Study the drawing (mm; zero at the part's minimum x, y, z) and answer. A direction names the side the tool comes from. Coordinates: 2 decimals unless noted, no trailing zeros. Order: outer loops, then holes, each group sorted by start corner. A loop starts at its lowest first (then second) coordinate and runs counter-clockwise, first axis right, second up. Notation, with made-up numbers: (-0.75, 68) -> (17.25, 68) arc R13 cw to (17.25, 90) -> close; hole circle Ø9 at (30, 30). An arc over 180 degrees is marked (long way). Answer in a Markdown table with one row per item. Add a question column.
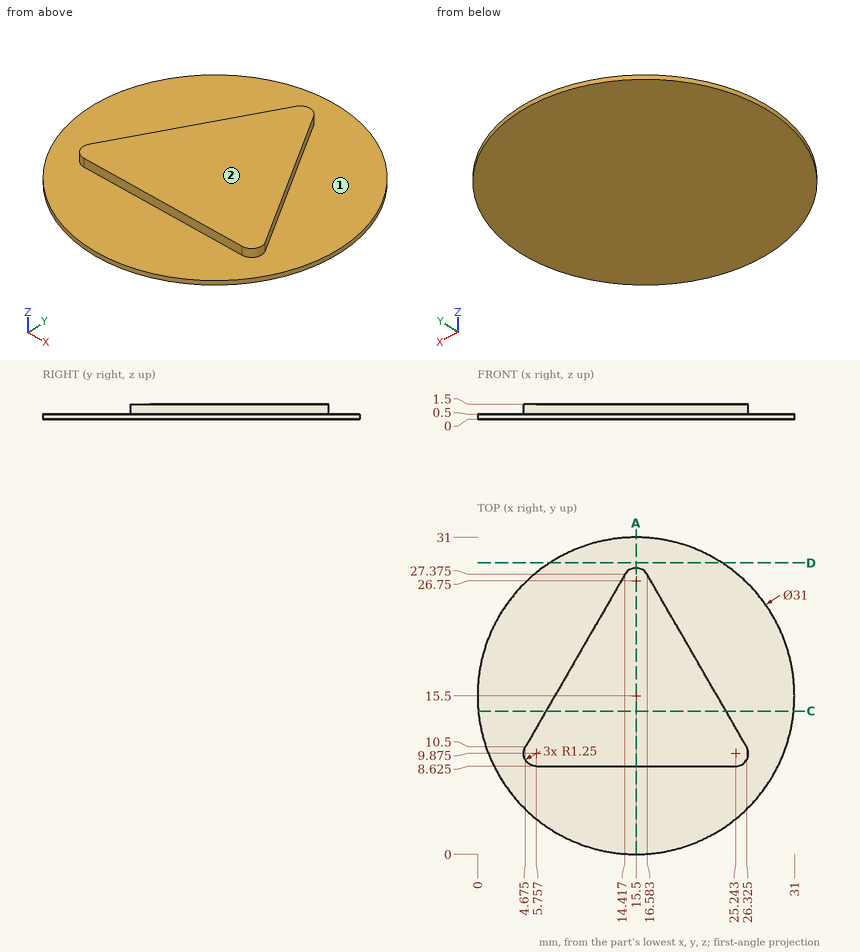
Q1. Straight lines are drawn through the part: line 1 (Z direction, x = 12.5, y = 4.5); line 2 (X direction, y = 10, z = 1); line 3 (Y direction, x = 11, z = 0.6) (1 decimal). For each, find the intervals that lie inside material, in ascending order.
Q2. A cutting plane is placed at A-A (x = 15.5). Determine the outline of the cut face in (y, z) (1 decimal).
Q3. Given pin 1 (0.8 mm diameter, centred on x = 12.5, z = 1, fed in from -Y) (3 decimals); pin 2 (4 mm diameter, centred on x = 25.5, y = 4.5, fed in from +Z), each flat-ended and moving along its own axis, determine where each tip first touches the part or whether it passes through.
Q4. A cutting plane is placed at D-D (y = 28.5). Determine the outline of the cut face in (x, z).
Q5. A cutting plane is placed at C-C (y = 14). Determine the outline of the cut face in (x, z) (1 decimal).
Q6. For the marked faces 1 and 2, determine the directions among +Z, -Z, +X, -X, +Y, -Y from which every point of the face is accessible in a straight line to the end or side of a thin tool.
Returned:
| question | item | result |
|---|---|---|
| 1 | line 1 | z = 0 to 0.5 |
| 1 | line 2 | x = 4.51 to 26.49 |
| 1 | line 3 | y = 8.6 to 21.5 |
| 2 | outline | (0, 0) -> (31, 0) -> (31, 0.5) -> (28, 0.5) -> (28, 1.5) -> (8.6, 1.5) -> (8.6, 0.5) -> (0, 0.5) -> close |
| 3 | pin 1 | stops at y = 8.625 |
| 3 | pin 2 | stops at z = 0.5 |
| 4 | outline | (7.06, 0) -> (23.94, 0) -> (23.94, 0.5) -> (7.06, 0.5) -> close |
| 5 | outline | (0.1, 0) -> (30.9, 0) -> (30.9, 0.5) -> (24.3, 0.5) -> (24.3, 1.5) -> (6.7, 1.5) -> (6.7, 0.5) -> (0.1, 0.5) -> close |
| 6 | face 1 | +Z |
| 6 | face 2 | +Z, +X, -X, +Y, -Y |
